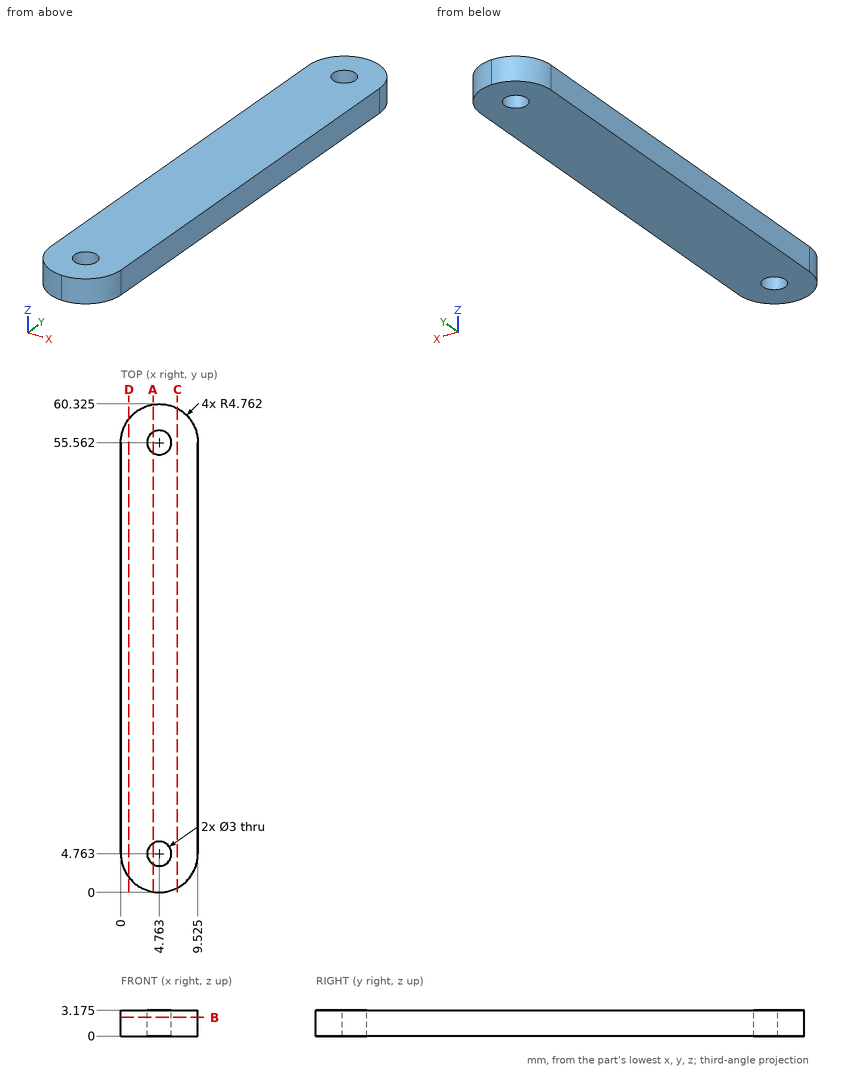
Part print with two shaded views. Sizes in mm from the minimum x, y, z corner. Round coordinates to 2 decimals unless told otherwise and drop trailing zeros. Loops run counter-clockwise (first coordinate to the right, second up) from the corner with the lowest first, then second, coordinate; pieces in that order, holes last. Notation, with made-up numbers: M -28.5,66 L -5.5,66 A28 cw -5.5,89 Z; hole C 64.25,81 d9. An arc over 180 degrees is marked long. Put each result on its own line as item: value. Start each with the question number.
Item 1: Cut at A-A (x = 4). List the corners of the cut face in (y, z) (1 decimal).
Item 2: Drill centre lines: line 1 along Y through (x, z) = (5.5, 0.8) (1 decimal); line 2 along Y through (x, z) = (5, 1.2) (1 decimal); line 3 along X through (y, z) = (4, 1.5) (1 decimal). Where is each one in solid material? Low to high.
Item 3: Cut at C-C (x = 7). List the corners of the cut face in (y, z) (1 decimal).
Item 4: Cut at D-D (x = 1). List the corners of the cut face in (y, z) (1 decimal), then the cut area to 3 significant figures.
Item 5: Cut at B-B (z = 2.3). Give the number of separate pieces and of enclosed holes in the cut face, then the cut area to 3 significant figures.
Answer block:
1. outline: M 0.1,0 L 3.5,0 L 3.5,3.2 L 0.1,3.2 Z; M 6.1,0 L 54.3,0 L 54.3,3.2 L 6.1,3.2 Z; M 56.9,0 L 60.3,0 L 60.3,3.2 L 56.9,3.2 Z
2. line 1: 0.1 to 3.5, 6.1 to 54.3, 56.9 to 60.3
2. line 2: 0 to 3.3, 6.2 to 54.1, 57 to 60.3
2. line 3: 0.1 to 3.5, 6.1 to 9.5
3. outline: M 0.6,0 L 59.8,0 L 59.8,3.2 L 0.6,3.2 Z
4. outline: M 1.8,0 L 58.5,0 L 58.5,3.2 L 1.8,3.2 Z
4. area: 180 mm2
5. separate pieces: 1
5. enclosed holes: 2
5. area: 541 mm2
